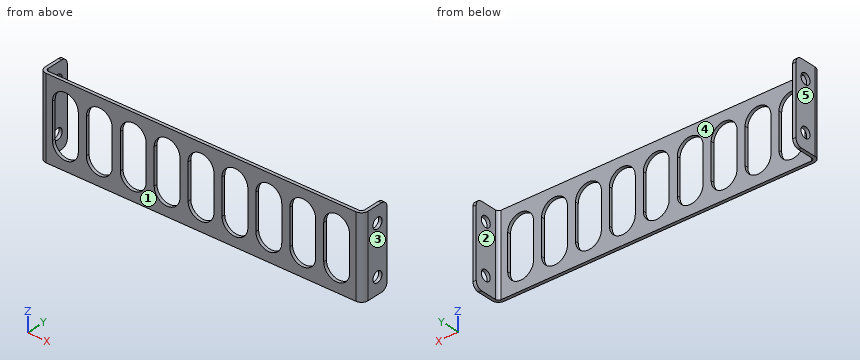
from build123d import *

# Parameters (mm, degrees)
SM_BASE_FLANGE_1_DEPTH   = 12.5
CUT_EXTRUDE_1_DEPTH      = 53.156015952
CUT_EXTRUDE_1_DEPTH_BACK = 53.156015952
SKETCH_6_R               = 1.65
CUT_EXTRUDE_2_DEPTH      = 10
FILLET_1_R               = 2


# Sheet-metal steps are written as plain solids
with BuildPart() as part:
    # Sketch 1 → 基体-法兰1 (new, symmetric)
    with BuildSketch(Plane.XY):
        with BuildLine():
            Line((-49, 8), (-49, 1))
            ThreePointArc((-49, 1), (-48.707106781, 0.292893219), (-48, 0))
            Line((-48, 0), (48, 0))
            ThreePointArc((48, 0), (48.707106781, 0.292893219), (49, 1))
            Line((49, 1), (49, 8))
            Line((49, 8), (50, 8))
            Line((50, 8), (50, 1))
            ThreePointArc((50, 1), (49.414213562, -0.414213562), (48, -1))
            Line((48, -1), (-48, -1))
            ThreePointArc((-48, -1), (-49.414213562, -0.414213562), (-50, 1))
            Line((-50, 1), (-50, 8))
            Line((-50, 8), (-49, 8))
        make_face()
    extrude(amount=SM_BASE_FLANGE_1_DEPTH, both=True)

    # 草图6 → 切除-拉伸1 (cut, two sides: drawn at the far end of the back side and taken through both)
    with BuildSketch(Plane(origin=(0, 0, 0), x_dir=(0, 0, -1), z_dir=(1, 0, 0)).offset(-CUT_EXTRUDE_1_DEPTH_BACK)):
        with Locations((-7.5, 4.5)):
            Circle(SKETCH_6_R)
        with Locations((7.5, 4.5)):
            Circle(SKETCH_6_R)
    extrude(amount=CUT_EXTRUDE_1_DEPTH + CUT_EXTRUDE_1_DEPTH_BACK, mode=Mode.SUBTRACT)

    # 草图7 → 切除-拉伸2 (cut)
    with BuildSketch(Plane.XZ.offset(1)):
        with BuildLine():
            Line((46, 5.5), (46, -5.5))
            ThreePointArc((46, -5.5), (42, -9.5), (38, -5.5))
            Line((38, -5.5), (38, 5.5))
            ThreePointArc((38, 5.5), (42, 9.5), (46, 5.5))
        make_face()
        with BuildLine():
            Line((-38, 5.5), (-38, -5.5))
            ThreePointArc((-38, -5.5), (-42, -9.5), (-46, -5.5))
            Line((-46, -5.5), (-46, 5.5))
            ThreePointArc((-46, 5.5), (-42, 9.5), (-38, 5.5))
        make_face()
        with BuildLine():
            Line((-27.5, 5.5), (-27.5, -5.5))
            ThreePointArc((-27.5, -5.5), (-31.5, -9.5), (-35.5, -5.5))
            Line((-35.5, -5.5), (-35.5, 5.5))
            ThreePointArc((-35.5, 5.5), (-31.5, 9.5), (-27.5, 5.5))
        make_face()
        with BuildLine():
            Line((-17, 5.5), (-17, -5.5))
            ThreePointArc((-17, -5.5), (-21, -9.5), (-25, -5.5))
            Line((-25, -5.5), (-25, 5.5))
            ThreePointArc((-25, 5.5), (-21, 9.5), (-17, 5.5))
        make_face()
        with BuildLine():
            Line((-6.5, 5.5), (-6.5, -5.5))
            ThreePointArc((-6.5, -5.5), (-10.5, -9.5), (-14.5, -5.5))
            Line((-14.5, -5.5), (-14.5, 5.5))
            ThreePointArc((-14.5, 5.5), (-10.5, 9.5), (-6.5, 5.5))
        make_face()
        with BuildLine():
            Line((4, 5.5), (4, -5.5))
            ThreePointArc((4, -5.5), (0, -9.5), (-4, -5.5))
            Line((-4, -5.5), (-4, 5.5))
            ThreePointArc((-4, 5.5), (0, 9.5), (4, 5.5))
        make_face()
        with BuildLine():
            Line((14.5, 5.5), (14.5, -5.5))
            ThreePointArc((14.5, -5.5), (10.5, -9.5), (6.5, -5.5))
            Line((6.5, -5.5), (6.5, 5.5))
            ThreePointArc((6.5, 5.5), (10.5, 9.5), (14.5, 5.5))
        make_face()
        with BuildLine():
            Line((25, 5.5), (25, -5.5))
            ThreePointArc((25, -5.5), (21, -9.5), (17, -5.5))
            Line((17, -5.5), (17, 5.5))
            ThreePointArc((17, 5.5), (21, 9.5), (25, 5.5))
        make_face()
        with BuildLine():
            Line((35.5, 5.5), (35.5, -5.5))
            ThreePointArc((35.5, -5.5), (31.5, -9.5), (27.5, -5.5))
            Line((27.5, -5.5), (27.5, 5.5))
            ThreePointArc((27.5, 5.5), (31.5, 9.5), (35.5, 5.5))
        make_face()
    extrude(amount=-CUT_EXTRUDE_2_DEPTH, mode=Mode.SUBTRACT)

    # 圆角1
    fillet_1_edges = [part.edges().sort_by_distance(p)[0] for p in [
        (-49.5, 8, -12.5),
        (49.5, 8, -12.5),
        (-49.5, 8, 12.5),
        (49.5, 8, 12.5),
    ]]
    fillet(fillet_1_edges, radius=FILLET_1_R)


solid = part.part
Design review of the part built by this model. Coordinates are the model's own, in mm. Face numbers are marked on the shaded views. A direction names the side the tool comes from. Coordinates: 2 decimals unless noted, no trailing zeros. Order: outer loops, then holes, each group sorted by start corner. A loop starts at its lowest first (then second) coordinate and runs counter-clockwise, first axis right, second up. Notation, with made-up numbers: M 15.25,50 L 52.25,50 A6 cw 52.25,59 Z; hole C 54.5,57.25 d9. An arc over 180 degrees is marked long. Use a Markdown table: item, result.
(1) Draft analysis for pull direction X (two halves, no side actions). For the marked faces 1, 2 and 3, state which applies: released by +X, released by -X, zero draft, split by the parting line, or undercut.
Worked answers:
| item | result |
|---|---|
| face 1 | zero draft |
| face 2 | undercut |
| face 3 | released by +X |
(2) For P1, Ø1.1, axis at y = -0.5, z = 0, coming from the -X side; P2, Ø0.5, axis at y = -0.5, z = -2.5, coming from the -X side; P3, Ø1.1, axis at y = -0.5, z = -2, coming from the +X side, all flat-tipped, find the tip position at first contact; note any pin that passes through.
Worked answers:
| item | result |
|---|---|
| P1 | stops at x = -49.76 |
| P2 | stops at x = -49.56 |
| P3 | stops at x = 49.76 |
(3) Add section A-A (x = 21). Give the boundary of the cut face in (y, z).
Worked answers:
| item | result |
|---|---|
| outline | M -1,-12.5 L 0,-12.5 L 0,-9.5 L -1,-9.5 Z; M -1,9.5 L 0,9.5 L 0,12.5 L -1,12.5 Z |
(4) Add section C-C (x = -43.5). Give the boundary of the cut face in (y, z).
Worked answers:
| item | result |
|---|---|
| outline | M -1,-12.5 L 0,-12.5 L 0,-9.21 L -1,-9.21 Z; M -1,9.21 L 0,9.21 L 0,12.5 L -1,12.5 Z |
(5) Wall thickness on probe 1 along Z at (x, y) = (-49.4, 4.5); probe 2 along X at (y, z) = (3, -4.5); probe 3 along X at (y, z) = (0.25, 7.5): over which ranges is each line inside the solid? List them lowest first.
Worked answers:
| item | result |
|---|---|
| probe 1 | z = -12.5 to -9.15, -5.85 to 5.85, 9.15 to 12.5 |
| probe 2 | x = -50 to -49, 49 to 50 |
| probe 3 | x = -49.85 to -48.66, 48.66 to 49.85 |
(6) Add section B-B (z = 3). Count the separate pieces of the cut face and the enclosed holes in it, then the cut area to 3 significant figures.
Worked answers:
| item | result |
|---|---|
| separate pieces | 10 |
| enclosed holes | 0 |
| area | 42.7 mm2 |
(7) For the marked faces 4 and 5, list the 3-axis set-ups (+Z, -Z, +X, -X, +Y, -Y) from which the entire face can be reached by the end or side of a thin tool; tool diameter is ignored.
Worked answers:
| item | result |
|---|---|
| face 4 | +Z, -Z, +Y |
| face 5 | +Z, -Z, -X, +Y, -Y |
